Source: CAD feature listing. Evaluate the final solid. Frame: model axes, mm. A direction names the side the tool comes from. Give positions to 0.01 mm unless a question says otherwise; leave off trailing zeros. Order: outer loops, then holes, each group sorted by start corner. A loop starts at its lowest first (then second) coordinate and runs counter-clockwise, first axis right, second up.
Autodesk Inventor part; units mm, degrees
ref_plane "YZ Plane" through (0, 0, 0) normal (1, 0, 0) x (0, 1, 0)
ref_plane "XZ Plane" through (0, 0, 0) normal (0, 1, 0) x (-1, 0, 0)
ref_plane "XY Plane" through (0, 0, 0) normal (0, 0, 1) x (1, 0, 0)
sketch "Sketch1" plane through (0, 0, 0) normal (0, 0, 1) x (1, 0, 0)
  line L0 (-198.755, 0) -> (114.6175, 0)
  line L1 (0, -97.79) -> (0, 97.79)
  circle A0 centre (0, 0) radius 50.8 construction
  arc A1 (-18.4326, -67.374) -> (-18.4326, 67.374) centre (0, 0) ccw
  arc A2 (44.9013, -44.9013) -> (44.9013, 44.9013) centre (0, 0) ccw
  arc A3 (40.1305, -40.1305) -> (40.1305, 40.1305) centre (0, 0) ccw
  line L2 (0, 0) -> (44.9013, 44.9013) construction
  line L3 (0, 0) -> (44.9013, -44.9013) construction
  arc A4 (44.9013, 44.9013) -> (40.1305, 40.1305) centre (42.5159, 42.5159) ccw
  arc A5 (40.1305, -40.1305) -> (44.9013, -44.9013) centre (42.5159, -42.5159) ccw
  circle A6 centre (-114.3, 0) radius 14.2875
  arc A7 (-124.7731, 38.2807) -> (-124.7731, -38.2807) centre (-114.3, 0) ccw
  line L4 (-114.3, -14.2875) -> (-114.3, 14.2875) construction
  line L5 (-124.7731, 38.2807) -> (-18.4326, 67.374)
  line L6 (-124.7731, -38.2807) -> (-18.4326, -67.374)
  circle A8 centre (-74.0404, 25.4) radius 11.1125
  circle A9 centre (-74.0404, -25.4) radius 11.1125
  circle A10 centre (0, 0) radius 19.05
  circle A11 centre (0, 0) radius 53.975
  dimension "d0" = 101.6
  dimension "d1" = 19.05
  dimension "d2" = 6.7469
  dimension "d3" = 6.35
  dimension "d6" = 28.575
  dimension "d7" = 25.4
  dimension "d9" = 22.225
  dimension "d10" = 38.1
  dimension "d11" = 45
  dimension "d12" = 45
  dimension "d13" = 3.175
  dimension "d14" = 114.3
extrude "Extrusion1" add sketch "Sketch1" along normal mid plane 6.35 contours A11 L1 A1 L0 A2 A4 A3 | L0 A3 A5 A2 A1 L1 A11 | A11 L0 A6 A7 L5 A1 L1 | L1 A1 L6 A7 L0 A6 A11
properties part number "back plate"
1) Draft query along X for faces 1 (the flat face through (-59, 6, -3.175)), 2 (the cylindrical face through (-85.142, 24.911, -0.044)), 3 (the flat face through (-72.347, -52.624, -0.044)). Return one class per face: +X half, -X half, draft (parallel to the pull), parting line (faces both ways), or undercut.
Report:
face 1: draft
face 2: undercut
face 3: -X half
2) Reachability of faces 4 (the cylindrical face through (63.496, 0.698, -0.044)), 5 (the flat face through (-72.347, 52.624, -0.044)) from +Z, -Z, +X, -X, +Y, -Y: full face, straight path, thin tool, end or side. Return the list, or none.
Report:
face 4: +Z, -Z
face 5: +Z, -Z, -X, +Y
3) Section query C-C, the plane z = 1.5. Count the separate pieces of the cut face and the enclosed holes in it, and give its area (3 significant figures).
Report:
separate pieces: 1
enclosed holes: 5
area: 11,900 mm2
4) Pin query (flat end, axial travel): pin 1 (3 mm diameter, centred on y = -10.5, z = -2, fed in from -X); pin 2 (17 mm diameter, centred on x = -114.3, y = 0, fed in from -Z); pin 3 (3 mm diameter, centred on y = -15.5, z = 2.5, fed in from -X); pin 4 (1 mm diameter, centred on y = -16.5, z = 1.5, fed in from -X). Return the tip coordinate at first contact, or that it passes through.
Report:
pin 1: stops at x = -152.95
pin 2: passes through
pin 3: stops at x = -151.44
pin 4: stops at x = -150.62
5) Section query B-B, the plane y = 0. Return the cut outline in (x, z) (1 decimal), and give its area (3 significant figures).
Report:
outline: (-154, -3.2) - (-128.6, -3.2) - (-128.6, 3.2) - (-154, 3.2) - close; (-100, -3.2) - (-54, -3.2) - (-54, 3.2) - (-100, 3.2) - close; (54, -3.2) - (56.8, -3.2) - (56.8, 3.2) - (54, 3.2) - close; (63.5, -3.2) - (69.8, -3.2) - (69.8, 3.2) - (63.5, 3.2) - close
area: 512 mm2
6) Section query A-A, the plane x = 0. Return the cut outline in (y, z) (3 decimals).
Report:
outline: (-69.85, -3.175) - (-53.975, -3.175) - (-53.975, 3.175) - (-69.85, 3.175) - close; (53.975, -3.175) - (69.85, -3.175) - (69.85, 3.175) - (53.975, 3.175) - close
7) Section query D-D, the plane x = -114.3. Return the cut outline in (y, z) (1 decimal).
Report:
outline: (-41.1, -3.2) - (-14.3, -3.2) - (-14.3, 3.2) - (-41.1, 3.2) - close; (14.3, -3.2) - (41.1, -3.2) - (41.1, 3.2) - (14.3, 3.2) - close
8) Material intervals for L1, parallel to X at y = 0, z = -0.5 (1 decimal); L2, parallel to Y at x = -2, z = 0.5; L3, parallel to X at y = 35.5, z = 0.5, sorted ascending.
Report:
L1: x = -154 to -128.6, -100 to -54, 54 to 56.8, 63.5 to 69.8
L2: y = -69.82 to -53.94, 53.94 to 69.82
L3: x = -132.04 to -78.67, -69.41 to -40.66, 40.66 to 44.28, 52.65 to 60.16
